Verification items for the finished model (mm, model axes). Face numbers are marked on the shaded views. A direction names the side the tool comes from. Give positions to 0.01 mm unless a question says otherwise; leave off trailing zeros. Order: outer loops, then holes, each group sorted by start corner. A loop starts at its lowest first (then second) coordinate and runs counter-clockwise, first axis right, second up.
from build123d import *
from build123d.topology import SkipClean

# Parameters (mm, degrees)
ESBO_O1_R                = 28
RESSALTO_EXTRUS_O1_DEPTH = 4
ESBO_O2_R                = 3
CORTE_EXTRUS_O1_DEPTH    = 40.799497484
PADR_OCIRCULAR1_COUNT    = 3
ESBO_O3_R                = 16.25
CORTE_EXTRUS_O2_DEPTH    = 40.799497484
RESSALTO_EXTRUS_O2_DEPTH = 13
PADR_OCIRCULAR2_COUNT    = 3
ESBO_O5_R                = 2.1
CORTE_EXTRUS_O3_DEPTH    = 8
PADR_OCIRCULAR3_COUNT    = 3
PADR_OCIRCULAR4_COUNT    = 3


with BuildPart() as part:
    # Esboço1 → Ressalto-extrusão1 (new body)
    with BuildSketch(Plane(origin=(0, 0, 0), x_dir=(1, 0, 0), z_dir=(0, 1, 0))):
        with Locations(Location((0, 0, 0), (0, 0, 270))):
            Circle(ESBO_O1_R)
    extrude(amount=RESSALTO_EXTRUS_O1_DEPTH)

    # Esboço2 → Corte-extrusão1 (cut, through all)
    with BuildSketch(Plane(origin=(0, 4, 0), x_dir=(1, 0, 0), z_dir=(0, 1, 0))):
        with Locations(Location((0, 22.5, 0), (0, 0, 270))):
            Circle(ESBO_O2_R)
    corte_extrus_o1 = extrude(amount=-CORTE_EXTRUS_O1_DEPTH, mode=Mode.SUBTRACT)

    # PadrãoCircular1: Corte-extrusão1 ×3 about axis
    padr_ocircular1_axis = Axis((0, 0, 0), (0, 1, 0))
    for i in range(1, PADR_OCIRCULAR1_COUNT):
        add(corte_extrus_o1.rotate(padr_ocircular1_axis, i * 360 / PADR_OCIRCULAR1_COUNT), mode=Mode.SUBTRACT)

    # Esboço3 → Corte-extrusão2 (cut, through all)
    with BuildSketch(Plane(origin=(0, 4, 0), x_dir=(1, 0, 0), z_dir=(0, 1, 0))):
        with Locations(Location((0, 0, 0), (0, 0, 270))):
            Circle(ESBO_O3_R)
    extrude(amount=-CORTE_EXTRUS_O2_DEPTH, mode=Mode.SUBTRACT)

    # Esboço4 → Ressalto-extrusão2 (add)
    with SkipClean():  # the faces are left unmerged after this step: merging them gives an invalid solid
        with BuildSketch(Plane(origin=(0, 4, 0), x_dir=(1, 0, 0), z_dir=(0, 1, 0))):
            with BuildLine():
                ThreePointArc((10.638713373, 12.283333333), (13.583103826, 16.7500617), (14.740590111, 21.973214286))
                ThreePointArc((14.740590111, 21.973214286), (15.299274914, 22.835165623), (16.322913343, 22.75))
                ThreePointArc((16.322913343, 22.75), (24.248711306, 14), (27.863534608, 2.761057619))
                ThreePointArc((27.863534608, 2.761057619), (27.425470986, 1.831977923), (26.39965683, 1.77911836))
                ThreePointArc((26.39965683, 1.77911836), (21.29753086, 3.388282126), (15.957035396, 3.071729378))
                ThreePointArc((15.957035396, 3.071729378), (14.072912811, 8.125), (10.638713373, 12.283333333))
            make_face()
        ressalto_extrus_o2 = extrude(amount=RESSALTO_EXTRUS_O2_DEPTH)

    # PadrãoCircular2: Ressalto-extrusão2 ×3 about axis
    with SkipClean():  # the faces are left unmerged after this step: merging them gives an invalid solid
        padr_ocircular2_axis = Axis((0, 0, 0), (0, 1, 0))
        for i in range(1, PADR_OCIRCULAR2_COUNT):
            add(ressalto_extrus_o2.rotate(padr_ocircular2_axis, i * 360 / PADR_OCIRCULAR2_COUNT))

    # Esboço5 → Corte-extrusão3 (cut)
    with SkipClean():  # the faces are left unmerged after this step: merging them gives an invalid solid
        with BuildSketch(Plane(origin=(0, 17, 0), x_dir=(1, 0, 0), z_dir=(0, 1, 0))):
            with Locations(Location((0, -22, 0), (0, 0, 270))):
                Circle(ESBO_O5_R)
        corte_extrus_o3 = extrude(amount=-CORTE_EXTRUS_O3_DEPTH, mode=Mode.SUBTRACT)

    # PadrãoCircular3: Corte-extrusão3 ×3 about axis
    with SkipClean():  # the faces are left unmerged after this step: merging them gives an invalid solid
        padr_ocircular3_axis = Axis((0, 0, 0), (0, 1, 0))
        for i in range(1, PADR_OCIRCULAR3_COUNT):
            add(corte_extrus_o3.rotate(padr_ocircular3_axis, i * 360 / PADR_OCIRCULAR3_COUNT), mode=Mode.SUBTRACT)

    # Loft1: read off the stored shape, not the designer's step
    # Loft1: loft between two sections, ruled curve by curve
    with SkipClean():  # the faces are left unmerged after this step: merging them gives an invalid solid
        loft1_from = [
            Edge.make_bspline([(7.471626812, 17, 24.108508402), (7.389968108, 17, 22.110176134), (5.391635839, 17, 22.191834838), (5.473294543, 17, 24.190167106), (5.554953247, 17, 26.188499375), (7.553285516, 17, 26.106840671), (7.471626812, 17, 24.108508402)], [0, 0, 0, 0, 0.5, 0.5, 0.5, 1, 1, 1, 1], 3, [1, 0.333333333, 0.333333333, 1, 0.333333333, 0.333333333, 1]),
        ]
        loft1_to = [
            Edge.make_bspline([(6.858825303, 19, 24.398982253), (7.358114301, 19, 23.626253002), (6.58538505, 19, 23.126964004), (6.086096051, 19, 23.899693255), (5.586807053, 19, 24.672422507), (6.359536305, 19, 25.171711505), (6.858825303, 19, 24.398982253)], [0, 0, 0, 0, 0.5, 0.5, 0.5, 1, 1, 1, 1], 3, [1, 0.333333333, 0.333333333, 1, 0.333333333, 0.333333333, 1]),
        ]
        loft1 = Solid(Shell([*[Face.make_surface_from_curves(loft1_from[k], loft1_to[k]) for k in range(1)], Face(Wire(loft1_from)), Face(Wire(loft1_to))]))
        add(loft1)

    # PadrãoCircular4: Loft1 ×3 about axis
    with SkipClean():  # the faces are left unmerged after this step: merging them gives an invalid solid
        padr_ocircular4_axis = Axis((0, 0, 0), (0, -1, 0))
        for i in range(1, PADR_OCIRCULAR4_COUNT):
            add(loft1.rotate(padr_ocircular4_axis, i * 360 / PADR_OCIRCULAR4_COUNT))


solid = part.part
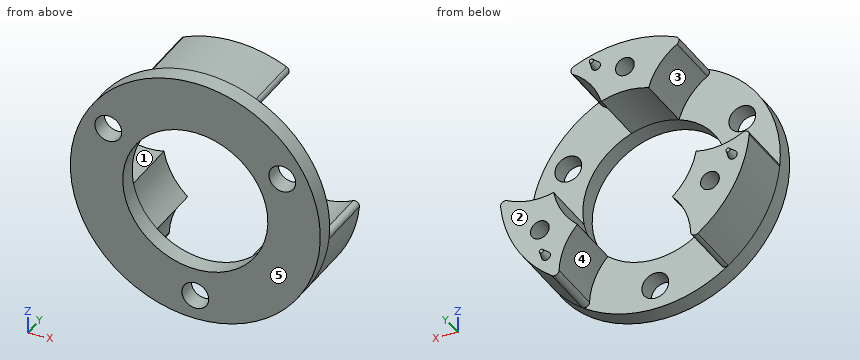
(1) Set-up check for the marked faces 4 and 5: record each of +Z, -Z, +X, -X, +Y, -Y from which the full face is reachable in a straight line by a thin tool's end or side.
Solved:
face 4: -Z, +Y
face 5: +Z, -Z, +X, -X, -Y
(2) Section check A-A, the plane y = 7.5. Enter the section's corners in (x, z).
Solved:
outline: (-27.86, -2.76) arc R28 ccw to (-16.32, -22.75) arc R1 ccw to (-14.74, -21.97) arc R14.75 cw to (-10.64, -12.28) arc R16.25 cw to (-15.96, -3.07) arc R14.75 cw to (-26.4, -1.78) arc R1 ccw to start; (-11.66, 23.75) arc R14.75 cw to (-5.32, 15.36) arc R16.25 cw to (5.32, 15.36) arc R14.75 cw to (11.66, 23.75) arc R1 ccw to (11.54, 25.51) arc R28 ccw to (-11.54, 25.51) arc R1 ccw to start; (10.64, -12.28) arc R14.75 cw to (14.74, -21.97) arc R1 ccw to (16.32, -22.75) arc R28 ccw to (27.86, -2.76) arc R1 ccw to (26.4, -1.78) arc R14.75 cw to (15.96, -3.07) arc R16.25 cw to start
(3) Go/stop test with flat-tipped pins: pin 1 (7 mm diameter, centred on x = -19.49, z = 11.25, fed in from -Y); pin 2 (4 mm diameter, centred on x = 19.05, z = -11, fed in from +Y); pin 3 (18 mm diameter, centred on x = -14, z = 8.5, fed in from +Y); pin 4 (2 mm diameter, centred on x = -21.5, y = 5, fed in from -Z). Record where each tip stops, or that it passes through.
Solved:
pin 1: stops at y = 0
pin 2: stops at y = 9
pin 3: stops at y = 4
pin 4: stops at z = -19.07
(4) Release check for a two-part mould opening along X. For the marked faces 1, 2 and 3 record: pulls with the +X half, pulls with the -X half, needs draft (parallel to the pull), parting line crosses it, or undercut.
Solved:
face 1: undercut
face 2: needs draft
face 3: pulls with the -X half
(5) Section check C-C, the plane z = -4.5. Enter the section's corners in (x, y).
Solved:
outline: (-27.64, 0) - (-15.61, 0) - (-15.61, 17) - (-27.64, 17) - close; (15.61, 0) - (27.64, 0) - (27.64, 17) - (15.61, 17) - close
(6) Section check B-B, the plane x = 0. Enter the section's corners in (y, z), then the cut area to 3 significant figures.
Solved:
outline: (0, -28) - (4, -28) - (4, -25.5) - (0, -25.5) - close; (0, -19.5) - (4, -19.5) - (4, -16.25) - (0, -16.25) - close; (0, 16.25) - (17, 16.25) - (17, 19.9) - (9, 19.9) - (9, 24.1) - (17, 24.1) - (17, 28) - (0, 28) - close
area: 189 mm2
(7) Section check D-D, the plane y = 12.5. Enter the section's corners in (x, z), then the cut area to 3 significant figures.
Solved:
outline: (-27.86, -2.76) arc R28 ccw to (-16.32, -22.75) arc R1 ccw to (-14.74, -21.97) arc R14.75 cw to (-10.64, -12.28) arc R16.25 cw to (-15.96, -3.07) arc R14.75 cw to (-26.4, -1.78) arc R1 ccw to start; (-11.66, 23.75) arc R14.75 cw to (-5.32, 15.36) arc R16.25 cw to (5.32, 15.36) arc R14.75 cw to (11.66, 23.75) arc R1 ccw to (11.54, 25.51) arc R28 ccw to (-11.54, 25.51) arc R1 ccw to start; (10.64, -12.28) arc R14.75 cw to (14.74, -21.97) arc R1 ccw to (16.32, -22.75) arc R28 ccw to (27.86, -2.76) arc R1 ccw to (26.4, -1.78) arc R14.75 cw to (15.96, -3.07) arc R16.25 cw to start; hole circle Ø4.2 at (-19.05, -11); hole circle Ø4.2 at (0, 22); hole circle Ø4.2 at (19.05, -11)
area: 568 mm2
(8) Scan lines: line 1 (X direction, y = 2.05, z = 11.25); line 2 (X direction, y = 12, z = -9.5); line 3 (Y direction, x = 23.5, z = 8). Record each from-to range of solid material in increasing order.
Solved:
line 1: x = -25.64 to -22.49, -16.49 to -11.73, 11.73 to 16.49, 22.49 to 25.64
line 2: x = -26.34 to -20.52, -17.58 to -13.18, 13.18 to 17.58, 20.52 to 26.34
line 3: y = 0 to 4
